The listing builds one solid part. Answer for the finished solid, in the listing's coordinates (mm). A direction names the side the tool comes from. Coordinates: 2 decimals unless noted, no trailing zeros. Order: outer loops, then holes, each group sorted by start corner. A loop starts at its lowest first (then second) coordinate and runs counter-clockwise, first axis right, second up. Notation, with made-up numbers: (64.25, 23.25) - (123.25, 23.25) arc R5 cw to (123.25, 29.25) - close; hole circle Ø2 at (38, 8.5). An arc over 180 degrees is marked (long way). Use a Markdown table: item, result. Add a question column.
Item 1: For faces 1 (the cylindrical face through (15.06, 51.25, -14.38)), 2 (the flat face through (11, 50, -14)), 3 (the flat face through (8, 23, -28.5)), determine the directions among +Z, -Z, +X, -X, +Y, -Y from which every point of the face is accessible in a straight line to the end or side of a thin tool.
Item 2: The part is cut by section C-C, the plane z = -20.5. Give the vertices of the cut face in (x, y), then the cut area to 3 significant figures.
Item 3: The part is cut by section B-B, the plane x = 3.25. Give the vertices of the cut face in (y, z).
Item 4: The part is cut by section A-A, the plane y = 5.25. Give the vertices of the cut face in (x, z) (3 decimals), then the cut area to 3 significant figures.
Item 5: Find the intervals of material crossed by line 1 along Y through (x, z) = (6, -29.7) (3 decimals); line 2 along Y through (x, z) = (10.5, -3.5); line 3 along X through (y, z) = (47.25, -22.25) (3 decimals), in increasing order.
Item 6: The part is cut by section D-D, the plane y = 35.25. Give the vertices of the cut face in (x, z).
Item 7: The mould has two halves that part along Z. Classify faces 4 (the flat face through (9, 23, 2)), 5 (the cylindrical face through (17.99, 26.6, -9.75)), 6 (the flat face through (7, 48.5, -14)): released by +Z, released by -Z, zero draft, split by the parting line, or undercut.
Item 8: Flat-ended cylindrical pins translate along their axes: P1, Ø8.5, axis at x = 9.5, z = -11, coming from the +Y side; P2, Ø1.8, axis at x = 6, z = -6.25, coming from the -Y side; P3, Ø3, axis at x = 9, z = -2.5, coming from the +Y side. Find the tip coordinate at first contact, or state that the pin passes through.
from build123d import *

# Parameters (mm, degrees)
SKETCH1_W                 = 32.5
SKETCH1_H                 = 50.5
SKETCH1_W_2               = 28.5
SKETCH1_H_2               = 46.5
EXTRUDE_THIN1_DEPTH       = 17
TAP_DRILL_FOR_M2_5_TAP1_D = 2.05
TAP_DRILL_FOR_M2_5_TAP2_D = 2.05
SKETCH7_W                 = 32.5
SKETCH7_H                 = 50.5
BOSS_EXTRUDE1_DEPTH       = 2
SKETCH9_R                 = 9.75
CUT_EXTRUDE1_DEPTH        = 2
BOSS_EXTRUDE2_DEPTH       = 8


with BuildPart() as part:
    # Sketch1 → Extrude-Thin1 (new body)
    with BuildSketch(Plane(origin=(0, 0, 0), x_dir=(0, 0, -1), z_dir=(1, 0, 0))):
        with Locations((14.25, 23.25)):
            Rectangle(SKETCH1_W, SKETCH1_H)
        with Locations((14.25, 23.25)):
            Rectangle(SKETCH1_W_2, SKETCH1_H_2, mode=Mode.SUBTRACT)
    extrude(amount=EXTRUDE_THIN1_DEPTH)

    # Tap Drill for M2.5 Tap1 (through all)
    with Locations(Plane(origin=(6, 29.25, 2), x_dir=(1, 0, 0), z_dir=(0, 0, 1))):
        with Locations((0, 0), (0, -24)):
            Hole(TAP_DRILL_FOR_M2_5_TAP1_D / 2)

    # Tap Drill for M2.5 Tap2 (through all)
    with Locations(Plane(origin=(6, 48.5, -6.25), x_dir=(0, 0, 1), z_dir=(0, 1, 0))):
        with Locations((0, 0), (-16, 0)):
            Hole(TAP_DRILL_FOR_M2_5_TAP2_D / 2)

    # Sketch7 → Boss-Extrude1 (add)
    with BuildSketch(Plane(origin=(17, 0, 0), x_dir=(0, 0, -1), z_dir=(1, 0, 0))):
        with Locations((14.25, 23.25)):
            Rectangle(SKETCH7_W, SKETCH7_H)
    extrude(amount=BOSS_EXTRUDE1_DEPTH)

    # Sketch9 → Cut-Extrude1 (cut)
    with BuildSketch(Plane.ZY.offset(-17)):
        with Locations((-14.25, 35.25)):
            Circle(SKETCH9_R)
    extrude(amount=-CUT_EXTRUDE1_DEPTH, mode=Mode.SUBTRACT)

    # Sketch10 → Boss-Extrude2 (add)
    with BuildSketch(Plane(origin=(19, 0, 0), x_dir=(0, 0, -1), z_dir=(1, 0, 0))):
        with BuildLine():
            Line((5.281304443, 48.5), (23.218695557, 48.5))
            ThreePointArc((23.218695557, 48.5), (14.25, 51.25), (5.281304443, 48.5))
        make_face()
    extrude(amount=-BOSS_EXTRUDE2_DEPTH)


solid = part.part
Solution:
| question | item | result |
|---|---|---|
| 1 | face 1 | +X, -X, +Y |
| 1 | face 2 | +Z, -Z, -X, +Y |
| 1 | face 3 | -X |
| 2 | outline | (0, -2) - (19, -2) - (19, 27.77) - (17, 27.77) - (17, 0) - (0, 0) - close; (0, 46.5) - (17, 46.5) - (17, 42.73) - (19, 42.73) - (19, 49.98) - (11, 49.98) - (11, 48.5) - (0, 48.5) - close |
| 2 | area | 151 mm2 |
| 3 | outline | (-2, -30.5) - (48.5, -30.5) - (48.5, 2) - (-2, 2) - close; hole (0, -28.5) - (46.5, -28.5) - (46.5, 0) - (0, 0) - close |
| 4 | outline | (0, -30.5) - (4.975, -30.5) - (4.975, -28.5) - (0, -28.5) - close; (0, 0) - (4.975, 0) - (4.975, 2) - (0, 2) - close; (7.025, -30.5) - (19, -30.5) - (19, 2) - (7.025, 2) - (7.025, 0) - (17, 0) - (17, -28.5) - (7.025, -28.5) - close |
| 4 | area | 125 mm2 |
| 5 | line 1 | y = -2 to 4.225, 6.275 to 28.225, 30.275 to 48.5 |
| 5 | line 2 | y = -2 to 0, 46.5 to 48.5 |
| 5 | line 3 | x = 0 to 4.975, 7.025 to 19 |
| 6 | outline | (0, -30.5) - (19, -30.5) - (19, -24) - (17, -24) - (17, -28.5) - (0, -28.5) - close; (0, 0) - (17, 0) - (17, -4.5) - (19, -4.5) - (19, 2) - (0, 2) - close |
| 7 | face 4 | released by +Z |
| 7 | face 5 | undercut |
| 7 | face 6 | zero draft |
| 8 | P1 | stops at y = 51.25 |
| 8 | P2 | passes through |
| 8 | P3 | stops at y = 48.5 |
